```python
from build123d import *

# Parameters (mm, degrees)
F0_R     = 304.8
F0_W     = 139.7
F0_H     = 139.7
F1_DEPTH = 406.4
F2_W     = 139.7
F2_H     = 139.7
F3_DEPTH = 203.2


with BuildPart() as f1:
    # F0 (on Top) → F1 (new body)
    with BuildSketch(Plane.XY):
        with Locations((-64.029319, 93.181163)):
            Circle(F0_R)
        with Locations((-64.029319, 93.181163)):
            Rectangle(F0_W, F0_H, mode=Mode.SUBTRACT)
    extrude(amount=F1_DEPTH)

    # F2 (on face) → F3 (join)
    with BuildSketch(Plane.XY.offset(406.4)):
        with Locations((-64.029319, 93.181163)):
            Rectangle(F2_W, F2_H)
    extrude(amount=-F3_DEPTH)


solid = f1.part
```
Check sheet for the modelled part. Datum: model origin and axes. Units: mm. A direction names the side the tool comes from. Give positions to 0.01 mm unless a question says otherwise; leave off trailing zeros. Write each loop counter-clockwise with the first axis right and the second up, starting at its lowest first coordinate (ties: lowest second). Pieces come first, ordered by that corner, then holes.
Item 1: Gauge pin test, flat ends, axial feed: pin 1 (12 mm diameter, centred on x = -146.5, z = 296.5, fed in from -Y); pin 2 (12 mm diameter, centred on x = -102.5, z = 253, fed in from -Y); pin 3 (6 mm diameter, centred on y = 129.5, z = 209.5, fed in from -X). Record the tip position at first contact, or that the pin passes through.
Item 2: Cross-section at B-B (z = 60). Enter the section's corners in (x, y), and give its area (3 significant figures).
Item 3: Cross-section at A-A (x = -72). Enter the section's corners in (y, z), and give its area (3 significant figures).
Item 4: Scan lines: L1, parallel to X at y = 87, z = 17; L2, parallel to X at y = 158, z = 202; L3, parallel to Y at x = -7.5, z = 182.5. Record each from-to range of solid material in increasing order.
Item 5: Draft check along X on faces 3 (the face through (-65, 94, 203.2)), 4 (the face through (-68, 165, 0)), 5 (the face through (-130.1, -204.37, 200.36)). Enter one of: released by +X, released by -X, zero draft, split by the parting line, or undercut.
Item 6: Cross-section at D-D (z = 292.5). Enter the section's corners in (x, y).
Item 7: Cross-section at C-C (y = 46.5). Enter the section's corners in (x, z).
Item 8: Access from +Z, -Z, +X, -X, +Y, -Y to the whole of each face (thin tool, end or side, straight path). Record for faces 1 (the face through (-68, 97, 406.4)), 2 (the face through (-65, 163.031, 100)).
Report:
1. pin 1: stops at y = -201.87
1. pin 2: stops at y = -209.88
1. pin 3: stops at x = -367
2. outline: circle Ø609.6 at (-64.03, 93.18); hole (-133.88, 23.33) - (5.82, 23.33) - (5.82, 163.03) - (-133.88, 163.03) - close
2. area: 272,000 mm2
3. outline: (-211.51, 0) - (23.33, 0) - (23.33, 203.2) - (163.03, 203.2) - (163.03, 0) - (397.88, 0) - (397.88, 406.4) - (-211.51, 406.4) - close
3. area: 219,000 mm2
4. L1: x = -368.77 to -133.88, 5.82 to 240.71
4. L2: x = -361.86 to -133.88, 5.82 to 233.8
4. L3: y = -206.33 to 23.33, 163.03 to 392.69
5. face 3: undercut
5. face 4: zero draft
5. face 5: split by the parting line
6. outline: circle Ø609.6 at (-64.03, 93.18)
7. outline: (-365.23, 0) - (-133.88, 0) - (-133.88, 203.2) - (5.82, 203.2) - (5.82, 0) - (237.17, 0) - (237.17, 406.4) - (-365.23, 406.4) - close
8. face 1: +Z, +X, -X, +Y, -Y
8. face 2: -Z
